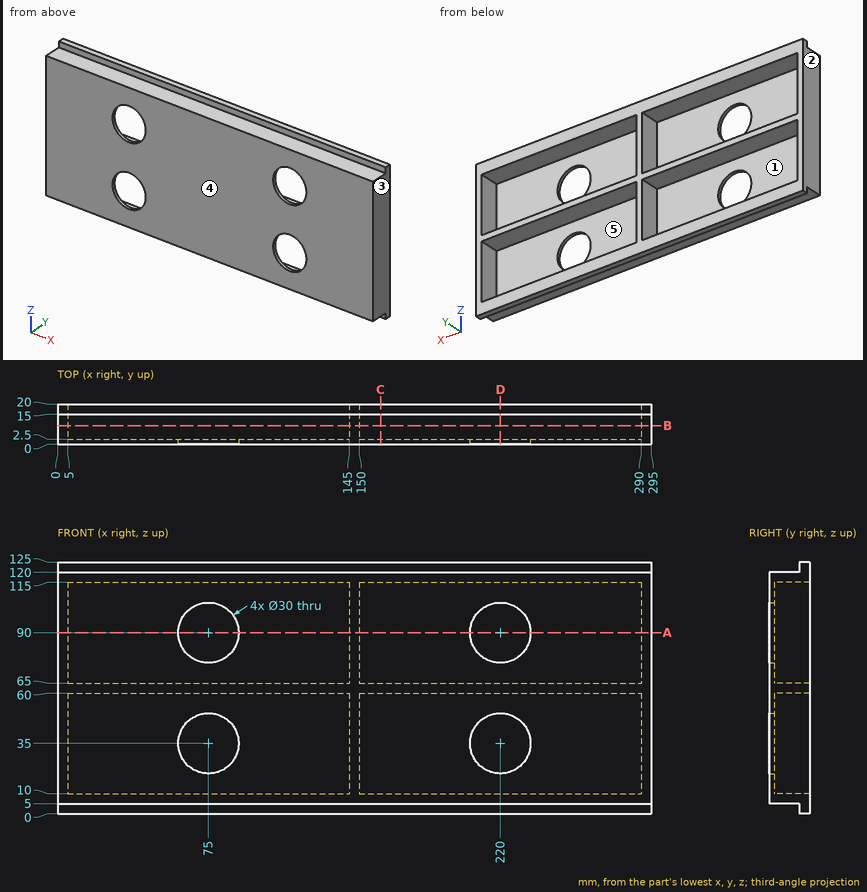
Job drawing, mm, ordinate dimensions from the low corner. One solid piece. A direction names the side the tool comes from. Coordinates: 2 decimals unless noted, no trailing zeros. Write each loop counter-clockwise with the first axis right and the second up, starting at its lowest first coordinate (ties: lowest second). Pieces come first, ordered by that corner, then holes.
Item 1: Slice it at A-A (z = 90). Write the cut outline in (x, y).
Item 2: Which spindle directions (+Z, -Z, +X, -X, +Y, -Y) get a long thin tool onto all of the face, cutting with end or side? Do the marked faces 4 and 5. Say none if no direction does.
Item 3: Slice it at C-C (x = 160.5). Write the cut outline in (y, z), and give its area (3 significant figures).
Item 4: Probe line 1 (Z direction, x = 134, y = 9); line 2 (X direction, y = 8.25, z = 51); line 3 (X direction, y = 0.75, z = 90). List the from-to ranges inside material, lowest first.
Item 5: Pin check, flat tips, straight feed: pin 1 (4 mm diameter, centred on x = 112, z = 29.5, fed in from +Y); pin 2 (4 mm diameter, centred on x = 181, y = 3, fed in from -Z); pin 3 (5 mm diameter, centred on x = 193.5, y = 11.5, fed in from +Z); pin 4 (18 mm diameter, centred on x = 75, z = 35, fed in from -Y). Stop position of each tip, or through.
Item 6: Slice it at D-D (x = 220). Write the cut outline in (y, z).
Item 7: Slice it at B-B (y = 9.25). Write the cut outline in (x, z), and give its area (4 significant figures).
Item 8: Mould opens along X. For the marked faces 1, 2 and 3 say: released by +X, released by -X, zero draft, split by the parting line, or undercut.
Results found:
1. outline: (0, 0) - (60, 0) - (60, 2.5) - (5, 2.5) - (5, 20) - (0, 20) - close; (90, 0) - (205, 0) - (205, 2.5) - (150, 2.5) - (150, 20) - (145, 20) - (145, 2.5) - (90, 2.5) - close; (235, 0) - (295, 0) - (295, 20) - (290, 20) - (290, 2.5) - (235, 2.5) - close
2. face 4: +Z, -Z, +X, -X, -Y
2. face 5: +Y
3. outline: (0, 5) - (15, 5) - (15, 0) - (20, 0) - (20, 10) - (2.5, 10) - (2.5, 60) - (20, 60) - (20, 65) - (2.5, 65) - (2.5, 115) - (20, 115) - (20, 125) - (15, 125) - (15, 120) - (0, 120) - close
3. area: 600 mm2
4. line 1: z = 5 to 10, 60 to 65, 115 to 120
4. line 2: x = 0 to 5, 145 to 150, 290 to 295
4. line 3: x = 0 to 60, 90 to 205, 235 to 295
5. pin 1: stops at y = 2.5
5. pin 2: stops at z = 5
5. pin 3: stops at z = 120
5. pin 4: passes through
6. outline: (0, 5) - (15, 5) - (15, 0) - (20, 0) - (20, 10) - (2.5, 10) - (2.5, 20) - (0, 20) - close; (0, 50) - (2.5, 50) - (2.5, 60) - (20, 60) - (20, 65) - (2.5, 65) - (2.5, 75) - (0, 75) - close; (0, 105) - (2.5, 105) - (2.5, 115) - (20, 115) - (20, 125) - (15, 125) - (15, 120) - (0, 120) - close
7. outline: (0, 5) - (295, 5) - (295, 120) - (0, 120) - close; hole (5, 10) - (145, 10) - (145, 60) - (5, 60) - close; hole (5, 65) - (145, 65) - (145, 115) - (5, 115) - close; hole (150, 10) - (290, 10) - (290, 60) - (150, 60) - close; hole (150, 65) - (290, 65) - (290, 115) - (150, 115) - close
7. area: 5,925 mm2
8. face 1: undercut
8. face 2: released by -X
8. face 3: released by +X
